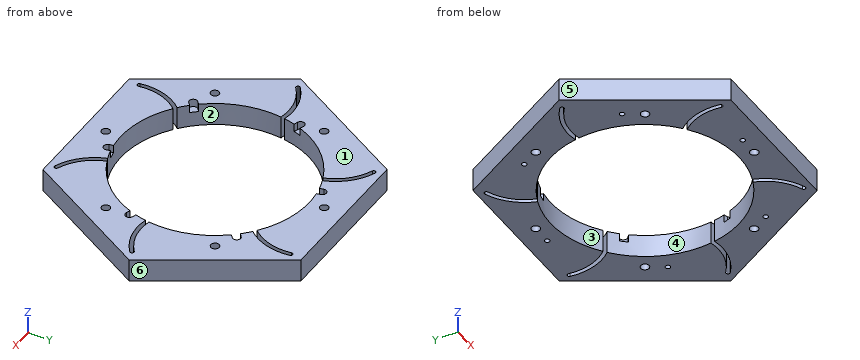
from build123d import *

# Parameters (mm, degrees)
F2_START      = 2
F0_R          = 4.2
F0_R_2        = 95
F2_DEPTH      = 23
F4_DEPTH      = 35
F4_DEPTH_BACK = 10
F5_COUNT      = 6
F8_DEPTH      = 8
F8_DEPTH_BACK = 10
F9_COUNT      = 6
F12_D         = 5
F12_DEPTH     = 12
F12_START     = 2
F12_TIP       = 1.5021515476


with BuildPart() as f2:
    # F0 (on Top) → F2 (new body)
    with BuildSketch(Plane.XY.offset(F2_START)):
        Polygon((75, 129.9038105677), (-75, 129.9038105677), (-150, 0), (-75, -129.9038105677), (75, -129.9038105677), (150, 0), align=None)
        with Locations((-95.2627944163, -55)):
            Circle(F0_R, mode=Mode.SUBTRACT)
        with Locations((0, -110)):
            Circle(F0_R, mode=Mode.SUBTRACT)
        with Locations((95.2627944163, -55)):
            Circle(F0_R, mode=Mode.SUBTRACT)
        with Locations((-95.2627944163, 55)):
            Circle(F0_R, mode=Mode.SUBTRACT)
        Circle(F0_R_2, mode=Mode.SUBTRACT)
        with Locations((95.2627944163, 55)):
            Circle(F0_R, mode=Mode.SUBTRACT)
        with Locations((0, 110)):
            Circle(F0_R, mode=Mode.SUBTRACT)
    extrude(amount=F2_DEPTH)


with BuildPart() as f4:
    # F3 (on Top) → F4 (new body, two sides)
    with BuildSketch(Plane.XY) as f4_sk:
        with BuildLine():
            ThreePointArc((-34.5435296861, 77.6643068393), (-32.6327882373, 78.4863117484), (-30.7025049427, 79.2613158498))
            ThreePointArc((-30.7025049427, 79.2613158498), (-41.9019572207, 106.1559598637), (-65.2675230757, 123.5571075336))
            ThreePointArc((-65.2675230757, 123.5571075336), (-66.656996648, 123.5810891624), (-67.7266746593, 122.6939584625))
            ThreePointArc((-67.7266746593, 122.6939584625), (-67.8817545517, 121.0315856662), (-66.7217246277, 119.8308093913))
            ThreePointArc((-66.7217246277, 119.8308093913), (-44.7195832857, 103.2599332678), (-34.5435296861, 77.6643068393))
        make_face()
    extrude(amount=F4_DEPTH)
    extrude(f4_sk.sketch, amount=-F4_DEPTH_BACK)


with BuildPart() as f5_1:
    # F5: instance of F4
    add(f4.part.rotate(Axis((0, 0, -0.1854561269), (0, 0, 1)), 1 * 360 / F5_COUNT))


with BuildPart() as f5_2:
    # F5: instance of F4
    add(f4.part.rotate(Axis((0, 0, -0.1854561269), (0, 0, 1)), 2 * 360 / F5_COUNT))


with BuildPart() as f5_3:
    # F5: instance of F4
    add(f4.part.rotate(Axis((0, 0, -0.1854561269), (0, 0, 1)), 3 * 360 / F5_COUNT))


with BuildPart() as f5_4:
    # F5: instance of F4
    add(f4.part.rotate(Axis((0, 0, -0.1854561269), (0, 0, 1)), 4 * 360 / F5_COUNT))


with BuildPart() as f5_5:
    # F5: instance of F4
    add(f4.part.rotate(Axis((0, 0, -0.1854561269), (0, 0, 1)), 5 * 360 / F5_COUNT))


with BuildPart() as f2_1:
    add(f2.part)

    # F6: cut F4, F5_5, F5_4, F5_3, F5_2, F5_1
    add(f4.part, mode=Mode.SUBTRACT)
    add(f5_5.part, mode=Mode.SUBTRACT)
    add(f5_4.part, mode=Mode.SUBTRACT)
    add(f5_3.part, mode=Mode.SUBTRACT)
    add(f5_2.part, mode=Mode.SUBTRACT)
    add(f5_1.part, mode=Mode.SUBTRACT)

    # F9: F8 ×6 about axis
    f9_axis = Axis((0, 0, -0.1854561269), (0, 0, 1))


with BuildPart() as f8:
    # F7 (on face) → F8 (new body, two sides)
    with BuildSketch(Plane.XY.offset(25)) as f8_sk:
        with BuildLine():
            ThreePointArc((-14.9635818085, 97.9443271428), (-16.6533189284, 100.4972414515), (-19.6533265238, 101.1075998951))
            ThreePointArc((-19.6533265238, 101.1075998951), (-22.2062408325, 99.4178627752), (-22.8165992761, 96.4178551798))
            Line((-22.8165992761, 96.4178551798), (-20.6971664161, 85.5143183486))
            Line((-20.6971664161, 85.5143183486), (-16.7706576823, 86.2775543301))
            Line((-16.7706576823, 86.2775543301), (-12.8441489485, 87.0407903117))
            Line((-12.8441489485, 87.0407903117), (-14.9635818085, 97.9443271428))
        make_face()
    extrude(amount=-F8_DEPTH)
    extrude(f8_sk.sketch, amount=F8_DEPTH_BACK)


with BuildPart() as f2_2:
    add(f2_1.part)
    for i in range(1, F9_COUNT):
        add(f8.part.rotate(f9_axis, i * 360 / F9_COUNT), mode=Mode.SUBTRACT)

    # F9#seed: cut F8
    add(f8.part, mode=Mode.SUBTRACT)

    # F12
    # its depths count from where the whole tool has entered the part; down to there all is cleared
    with Locations(Plane(origin=(0, 0, 0), x_dir=(1, 0, 0), z_dir=(0, 0, -1)).offset(-F12_START)):
        with Locations((-85.2627944163, -72.3205080757), (20, -110), (105.2627944163, -37.6794919243), (85.2627944163, 72.3205080757), (-20, 110), (-105.2627944163, 37.6794919243)):
            Hole(F12_D / 2, depth=F12_DEPTH)
            with Locations((0, 0, -(F12_DEPTH + F12_TIP / 2))):  # 118° drill point
                Cone(0, F12_D / 2, F12_TIP, mode=Mode.SUBTRACT)


solid = f2_2.part
Design review of the part built by this model. Coordinates are the model's own, in mm. Face numbers are marked on the shaded views. A direction names the side the tool comes from. Give positions to 0.01 mm unless a question says otherwise; leave off trailing zeros. Order: outer loops, then holes, each group sorted by start corner. A loop starts at its lowest first (then second) coordinate and runs counter-clockwise, first axis right, second up.
1. Tool access review of the marked faces 1 and 2: name each direction out of +Z, -Z, +X, -X, +Y, -Y from which nothing blocks a thin tool from reaching the whole face with its end or side.
Solution:
face 1: +Z, +X, -X, +Y, -Y
face 2: +Z, -Z
2. Add section B-B, the plane y = -55. State the section outline as (x, z) points.
Solution:
outline: (-118.25, 2) - (-99.46, 2) - (-99.46, 25) - (-118.25, 25) - close; (-91.06, 2) - (-77.46, 2) - (-77.46, 25) - (-91.06, 25) - close; (77.46, 2) - (91.06, 2) - (91.06, 25) - (77.46, 25) - close; (99.46, 2) - (118.25, 2) - (118.25, 25) - (99.46, 25) - close
3. Mouldability with a two-part tool opening along X and no side actions: class the marked faces 3, 4, 5 and 6 as +X half, -X half, draft (parallel to the pull), parting line (faces both ways), or undercut.
Solution:
face 3: undercut
face 4: undercut
face 5: -X half
face 6: +X half
4. Add section A-A, the plane x = 0. State the section outline as (y, z) points, then the cut area to 3 significant figures.
Solution:
outline: (-129.9, 2) - (-114.2, 2) - (-114.2, 25) - (-129.9, 25) - close; (-105.8, 2) - (-95, 2) - (-95, 25) - (-105.8, 25) - close; (95, 2) - (105.8, 2) - (105.8, 25) - (95, 25) - close; (114.2, 2) - (129.9, 2) - (129.9, 25) - (114.2, 25) - close
area: 1,220 mm2
5. To check wall thickness, follow L1, parallel to X at y = 67, z = 23; L2, parallel to X at y = 87.5, z = 14.5; L3, parallel to Y at x = 40, z = 23. State the ranges of each line that lie inside material, in increasing order.
Solution:
L1: x = -111.32 to -67.35, 67.35 to 70.98, 78.15 to 111.32
L2: x = -99.48 to -37, 37 to 65.77, 70.19 to 99.48
L3: y = -129.9 to -103.57, -95.82 to -86.17, 86.17 to 129.9
6. Add section C-C, the plane x = -125. State the section outline as (y, z) points, then the cut area to 3 significant figures.
Solution:
outline: (-43.3, 2) - (9.35, 2) - (9.35, 25) - (-43.3, 25) - close; (13.66, 2) - (43.3, 2) - (43.3, 25) - (13.66, 25) - close
area: 1,890 mm2
7. For pin 1 Ø3 at (x, y) = (-75.5, -64) entering from +Z; pin 2 Ø1 at (y, z) = (-34.5, 21) entering from +X; pin 3 Ø12 at (y, z) = (-79.5, 11.5) entering from -X, all flat-tipped, find the tip position at first contact; note any pin that passes through.
Solution:
pin 1: stops at z = 17
pin 2: stops at x = 130.37
pin 3: stops at x = -107.56
